The listing builds one solid part. Answer for the finished solid, in the listing's coordinates (mm). Face numbers are marked on the shaded views. Coordinates: 2 decimals unless noted, no trailing zeros. Order: outer loops, then holes, each group sorted by start corner. A loop starts at its lowest first (then second) coordinate and runs counter-clockwise, first axis right, second up. Notation, with made-up numbers: (66.5, 55.5) -> (99.5, 55.5) arc R34 ccw to (99.5, 90.5) -> close; hole circle Ø6 at (-28, 61.5). An arc over 180 degrees is marked (long way). Put each result on its own line as item: value. Start each with the question number.
```python
from build123d import *

# Parameters (mm, degrees)
SKETCH1_R                = 25
BOSS_EXTRUDE1_DEPTH      = 500
BOSS_EXTRUDE2_DEPTH      = 50
BOSS_EXTRUDE3_DEPTH      = 50
BOSS_EXTRUDE5_DEPTH      = 20
BOSS_EXTRUDE5_DEPTH_BACK = 55.4
SKETCH5_R                = 15
SKETCH8_R                = 24.878201485
BOSS_EXTRUDE6_DEPTH      = 500


with BuildPart() as part:
    # Sketch1 → Boss-Extrude1 (new body)
    with BuildSketch(Plane(origin=(0, 0, 0), x_dir=(1, 0, 0), z_dir=(0, 1, 0))):
        with Locations(Location((-21.996605786, 2.223061223, 0), (0, 0, 270))):
            Circle(SKETCH1_R)
    extrude(amount=BOSS_EXTRUDE1_DEPTH)

    # Sketch3 → Boss-Extrude2 (add)
    with BuildSketch(Plane(origin=(0, 500, 0), x_dir=(1, 0, 0), z_dir=(0, 1, 0))):
        Polygon((-46.996605786, 2.223061223), (-21.996605786, -22.776938777), (2.944600987, 2.164267995), (-22.055399013, 27.164267995), align=None)
    extrude(amount=BOSS_EXTRUDE2_DEPTH)

    # Sketch4 → Boss-Extrude3 (add)
    with BuildSketch(Plane(origin=(0, 0, 0), x_dir=(-1, 0, 0), z_dir=(0, -1, 0))):
        Polygon((46.996605786, 2.223061223), (21.996605786, 27.223061223), (-3.010340521, 2.216114917), (21.989659479, -22.783885083), align=None)
    extrude(amount=BOSS_EXTRUDE3_DEPTH)

    # Sketch5 → Boss-Extrude5 (add, two sides: drawn at the far end of the back side and taken through both)
    with BuildSketch(Plane(origin=(0.397112802, 0, 0.397112802), x_dir=(0.7071067811865474, 0, -0.7071067811865477), z_dir=(0.7071067811865477, 0, 0.7071067811865474)).offset(-BOSS_EXTRUDE5_DEPTH_BACK)):
        with Locations((-13.981523689, -31.399998411)):
            Circle(SKETCH5_R)
        with Locations((-14.023580538, 525)):
            Circle(SKETCH5_R)
    extrude(amount=BOSS_EXTRUDE5_DEPTH + BOSS_EXTRUDE5_DEPTH_BACK)

    # Sketch8 → Boss-Extrude6 (add)
    with BuildSketch(Plane(origin=(0, 550, 0), x_dir=(1, 0, 0), z_dir=(0, 1, 0))):
        with Locations(Location((-21.996605786, 2.223061223, 0), (0, 0, 89.990298588))):
            Circle(SKETCH8_R)
    extrude(amount=BOSS_EXTRUDE6_DEPTH)


solid = part.part
```
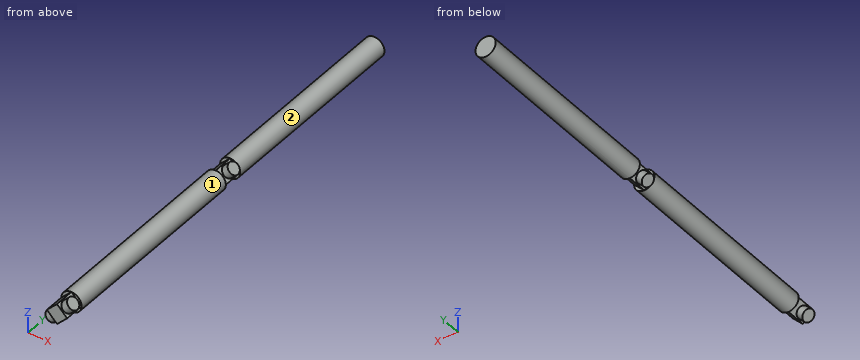
(1) For a pull along Y with two mould halves and no side action, classify the marked faces 1 and 2 as released by +Y, released by -Y, zero draft, split by the parting line, or undercut.
(2) Each of these flat-tipped pins is pushed along its axis until it touches: P1, Ø12, axis at y = 492.5, z = 8.5, coming from the -X side; P2, Ø3, axis at y = 707, z = -1, coming from the +X side; P3, Ø7.5, axis at x = -3.5, z = 15, coming from the -Y side; P4, Ø1, axis at x = -4, z = -21.5, coming from the -Y side. Where does it stop, or does it pass through?
(3) The part is cut by section B-B on y = 303. Determine the outline of the cut face in (x, z).
(4) The part is cut by section A-A on y = 916. Determine the outline of the cut face in (x, z), plus the area to 3 significant figures.
(5) Find the intervals of material crossed by L1, parallel to Y at x = -39, z = -19; L2, parallel to Y at x = -7.5, z = -19; L3, parallel to Y at x = -44.5, z = -6, in increasing order.
Worked out:
1. face 1: undercut
1. face 2: zero draft
2. P1: x = -46.55
2. P2: x = 2.88
2. P3: y = -46.4
2. P4: through
3. outline: circle Ø50 at (-22, -2.22)
4. outline: circle Ø49.76 at (-22, -2.22)
4. area: 1,940 mm2
5. L1: -46.4 to -16.4, 0 to 500, 510 to 540, 550 to 1050
5. L2: 0 to 500, 550 to 1050
5. L3: -38.45 to -24.35, 0 to 500, 517.88 to 532.12, 550 to 1050
